The listing builds one solid part. Answer for the finished solid, in the listing's coordinates (mm). A direction names the side the tool comes from. Round coordinates to 2 decimals unless told otherwise and drop trailing zeros. Loops run counter-clockwise (first coordinate to the right, second up) from the corner with the lowest first, then second, coordinate; pieces in that order, holes last. Notation, with made-up numbers: (31.5, 6) -> (79.5, 6) arc R32 cw to (79.5, 44) -> close; hole circle Ø11 at (84.25, 3). An arc over 180 degrees is marked (long way). Answer in a Markdown table with one row per item. Add a question column.
Autodesk Inventor part; units mm, degrees
ref_plane "YZ Plane" through (0, 0, 0) normal (1, 0, 0) x (0, 1, 0)
ref_plane "XZ Plane" through (0, 0, 0) normal (0, 1, 0) x (-1, 0, 0)
ref_plane "XY Plane" through (0, 0, 0) normal (0, 0, 1) x (1, 0, 0)
sketch "Sketch1" plane through (0, 0, 0) normal (0, 1, 0) x (-1, 0, 0)
  circle A0 centre (0, 0) radius 5
  line L0 (0, 0) -> (0, -40)
  circle A1 centre (0, -40) radius 1.75
  circle A2 centre (0, -40) radius 2.5
  line L1 (0, -40) -> (2.5, -40)
  line L2 (0, 0) -> (5, 0)
  line L3 (5, 0) -> (2.5, -40)
  line L4 (0, 0) -> (-5, 0)
  line L5 (0, -40) -> (-2.5, -40)
  line L6 (-5, 0) -> (-2.5, -40)
  dimension "d0" = 10
  dimension "d1" = 40
  dimension "d2" = 3.5
  dimension "d3" = 5
extrude "Extrusion1" add sketch "Sketch1" along normal blind 3 contours L2 L4 A0 | L3 A0 L0 L2 | L4 L0 A0 L6 | L3 A2 L0 A0 | A0 L0 A2 L6 | L1 A1 L0 A2 | A2 L5 A1 L1 | A2 L0 A1 L5 | L1 L0 A1 | A1 L5 L1 | A1 L0 L5
sketch "Sketch2" plane through (0, 3, 0) normal (0, 1, 0) x (1, 0, 0)
  arc A0 (2.5, 40) -> (-2.5, 40) centre (0, 40) ccw
  circle A1 centre (0, 40) radius 1.75
  point P0 (0, 0)
  dimension "d6" = 3.5
extrude "Extrusion2" cut sketch "Sketch2" against normal blind 5
sketch "Sketch4" plane through (0, 0, 0) normal (0, -1, 0) x (1, 0, 0)
  circle A0 centre (0, 0) radius 4
  line L0 (0, 0) -> (0, -14.45)
  circle A1 centre (0, -14.45) radius 2.5
  line L1 (0, 0) -> (-4, 0)
  line L2 (0, -14.45) -> (-2.5, -14.45)
  line L3 (0, -14.45) -> (2.5, -14.45)
  line L4 (0, 0) -> (4, 0)
  line L5 (2.5, -14.45) -> (13.578, -14.45) construction
  line L6 (2.5, -14.45) -> (3.0315, -2.6097)
  line L7 (2.5, -14.45) -> (14.3523, -14.45) construction
  line L8 (-2.5, -14.45) -> (-3.0325, -2.6084)
  line L9 (-2.5, -14.45) -> (9.3536, -14.45) construction
  dimension "d12" = 8
  dimension "d13" = 14.45
  dimension "d14" = 5
  dimension "d16" = 87.43
  dimension "d17" = 92.575
extrude "Extrusion4" cut sketch "Sketch4" against normal blind 1.5
sketch "Sketch5" plane through (0, 1.5, 0) normal (0, -1, 0) x (1, 0, 0)
  line L0 (0, 0) -> (0, -14.45)
  circle A0 centre (0, -14.45) radius 0.5
  line L1 (0, -14.45) -> (0, -12.45)
  circle A1 centre (0, -12.45) radius 0.5
  dimension "d20" = 14.45
  dimension "d21" = 1
  dimension "d24" = 2
  dimension "d25" = 1
extrude "Extrusion6" cut sketch "Sketch5" against normal blind 5
sketch "Sketch6" plane through (0, 1.5, 0) normal (0, -1, 0) x (1, 0, 0)
  arc A0 (3.0315, -2.6097) -> (-3.0325, -2.6084) centre (0, 0) ccw
  circle A1 centre (0, 0) radius 1
  point P0 (0, 0)
  dimension "d28" = 2
extrude "Extrusion7" cut sketch "Sketch6" against normal blind 2
properties part number "Servo_Arm"
Item 1: Section A-A, the plane x = 0 is taken. Write down the section's boundary in (y, z), and give its area (3 significant figures).
Item 2: The mould has two halves that part along Z. Classify faces 3 (the cylindrical face through (0.231, 2.24, -14.894)), 4 (the cylindrical face through (0, 1, 5)), 5 (the flat face through (0.1, 3, -13.1)): +Z half, -Z half, draft (parallel to the pull), parting line (faces both ways), or undercut.
Item 3: Consider L1, parallel to Z at x = 0, y = 2.7; L2, parallel to X at y = 1, z = 0; L3, parallel to Y at x = 1.5, z = -14. Determine where each line is inside the solid, lowest interval first. Write a range as from..to.
Item 4: Section D-D, the plane z = -3 is taken. Write down the section's boundary in (x, y), and give its area (3 significant figures).
Item 5: For faces 1 (the cylindrical face through (-0.1, 1.5, -42.5)), 2 (the flat face through (0, 1.5, -6)), determine the directions among +Z, -Z, +X, -X, +Y, -Y from which every point of the face is accessible in a straight line to the end or side of a thin tool.
Item 6: Flat-ended cylindrical pins translate along their axes: P1, Ø5, axis at x = 0, z = 0, coming from the -Y side; P2, Ø1, axis at y = 1, z = -19, coming from the +X side; P3, Ø1, axis at x = 1, y = 2.5, coming from the -Z side. Find the tip coordinate at first contact, or state that the pin passes through.
Item 7: Section B-B, the plane y = 1.95 is taken. Write down the section's boundary in (x, z).
Item 8: Section C-C, the plane z = -12.45 is taken. Write down the section's boundary in (x, y).
Here are the results:
| question | item | result |
|---|---|---|
| 1 | outline | (0, -42.5) -> (3, -42.5) -> (3, -41.75) -> (0, -41.75) -> close; (0, -38.25) -> (3, -38.25) -> (3, -14.95) -> (1.5, -14.95) -> (1.5, -16.95) -> (0, -16.95) -> close; (0, 4) -> (1.5, 4) -> (1.5, 1) -> (3, 1) -> (3, 5) -> (0, 5) -> close; (1.5, -13.95) -> (3, -13.95) -> (3, -12.95) -> (1.5, -12.95) -> close; (1.5, -11.95) -> (3, -11.95) -> (3, -1) -> (1.5, -1) -> close |
| 1 | area | 94.6 mm² |
| 2 | face 3 | undercut |
| 2 | face 4 | +Z half |
| 2 | face 5 | draft |
| 3 | L1 | z = -42.5..-41.75, -38.25..-14.95, -13.95..-12.95, -11.95..-1, 1..5 |
| 3 | L2 | x = -5..-4, 4..5 |
| 3 | L3 | y = 1.5..3 |
| 4 | outline | (-4.81, 0) -> (-3.01, 0) -> (-3.01, 1.5) -> (3.01, 1.5) -> (3.01, 0) -> (4.81, 0) -> (4.81, 3) -> (-4.81, 3) -> close |
| 4 | area | 19.8 mm² |
| 5 | face 1 | -Z, +Y, -Y |
| 5 | face 2 | -Y |
| 6 | P1 | stops at y = 1.5 |
| 6 | P2 | stops at x = 3.84 |
| 6 | P3 | stops at z = -42.45 |
| 7 | outline | (-5, 0) -> (-2.5, -40) arc R2.5 ccw to (2.5, -40) -> (5, 0) arc R5 ccw to start; hole circle Ø3.5 at (0, -40); hole circle Ø2 at (0, 0); hole circle Ø1 at (0, -14.45); hole circle Ø1 at (0, -12.45) |
| 8 | outline | (-4.22, 0) -> (-2.59, 0) -> (-2.59, 1.5) -> (-0.5, 1.5) -> (-0.5, 3) -> (-4.22, 3) -> close; (0.5, 1.5) -> (2.59, 1.5) -> (2.59, 0) -> (4.22, 0) -> (4.22, 3) -> (0.5, 3) -> close |
